Autodesk Inventor part; units mm, degrees
ref_plane "YZ Plane" through (0, 0, 0) normal (1, 0, 0) x (0, 1, 0)
ref_plane "XZ Plane" through (0, 0, 0) normal (0, 1, 0) x (-1, 0, 0)
ref_plane "XY Plane" through (0, 0, 0) normal (0, 0, 1) x (1, 0, 0)
sketch "Sketch1" plane through (0, 0, 0) normal (0, 0, 1) x (1, 0, 0)
  line L0 (-6, 110.6647) -> (-6, 110.2647)
  arc A0 (-6, 110.2647) -> (-5.6, 109.8647) centre (-5.6, 110.2647) ccw
  line L1 (-5.6, 109.8647) -> (-4.9, 109.8647)
  arc A1 (-4.9, 109.8647) -> (-4.7, 110.0647) centre (-4.9, 110.0647) ccw
  line L2 (-4.7, 110.0647) -> (-4.7, 110.3147)
  arc A2 (-4.5, 110.5147) -> (-4.7, 110.3147) centre (-4.5, 110.3147) ccw
  line L3 (-4.5, 110.5147) -> (-1.8, 110.5147)
  arc A3 (-1.4, 110.1147) -> (-1.8, 110.5147) centre (-1.8, 110.1147) ccw
  line L4 (-1.4, 110.1147) -> (-1.4, 104.4147)
  line L5 (-1.8, 104.0147) -> (-4.5, 104.0147)
  arc A4 (-1.8, 104.0147) -> (-1.4, 104.4147) centre (-1.8, 104.4147) ccw
  arc A5 (-4.7, 104.2147) -> (-4.5, 104.0147) centre (-4.5, 104.2147) ccw
  line L6 (-4.7, 104.2147) -> (-4.7, 104.4647)
  arc A6 (-4.7, 104.4647) -> (-4.9, 104.6647) centre (-4.9, 104.4647) ccw
  line L7 (-4.9, 104.6647) -> (-5.6, 104.6647)
  arc A7 (-5.6, 104.6647) -> (-6, 104.2647) centre (-5.6, 104.2647) ccw
  line L8 (-6, 104.2647) -> (-6, 103.6647)
  line L9 (-6.5, 116.6647) -> (-6.5, 110.6647)
  line L10 (-6.5, 110.6647) -> (-2.5, 110.6647)
  line L11 (-1.05, 103.6647) -> (-6.5, 103.6647)
  line L12 (-6.5, 103.6647) -> (-6.5, 97.1647)
  line L13 (-6.5, 97.1647) -> (-1.05, 97.1647)
  line L14 (-6, 97.1647) -> (-6, 96.5647)
  arc A8 (-6, 96.5647) -> (-5.6, 96.1647) centre (-5.6, 96.5647) ccw
  line L15 (-5.6, 96.1647) -> (-4.9, 96.1647)
  arc A9 (-4.9, 96.1647) -> (-4.7, 96.3647) centre (-4.9, 96.3647) ccw
  arc A10 (-4.5, 96.8147) -> (-4.7, 96.6147) centre (-4.5, 96.6147) ccw
  line L16 (-4.7, 96.3647) -> (-4.7, 96.6147)
  line L17 (-4.5, 96.8147) -> (-1.8, 96.8147)
  arc A11 (-1.4, 96.4147) -> (-1.8, 96.8147) centre (-1.8, 96.4147) ccw
  line L18 (-1.4, 96.4147) -> (-1.4, 90.7147)
  arc A12 (-1.8, 90.3147) -> (-1.4, 90.7147) centre (-1.8, 90.7147) ccw
  line L19 (-1.8, 90.3147) -> (-4.5, 90.3147)
  arc A13 (-4.7, 90.5147) -> (-4.5, 90.3147) centre (-4.5, 90.5147) ccw
  line L20 (-4.7, 90.5147) -> (-4.7, 90.7647)
  arc A14 (-4.7, 90.7647) -> (-4.9, 90.9647) centre (-4.9, 90.7647) ccw
  line L21 (-4.9, 90.9647) -> (-5.6, 90.9647)
  arc A15 (-5.6, 90.9647) -> (-6, 90.5647) centre (-5.6, 90.5647) ccw
  line L22 (-6, 90.5647) -> (-6, 90.1647)
  line L23 (-2.5, 90.1647) -> (-6.5, 90.1647)
  line L24 (-6.5, 90.1647) -> (-6.5, 84.1647)
  line L25 (32.5, 123.1647) -> (0, 123.1647)
  circle A16 centre (0, 116.6647) radius 4.75
  circle A17 centre (32.5, 116.6647) radius 4.75
  circle A18 centre (0, 84.1647) radius 4.75
  circle A19 centre (32.5, 84.1647) radius 4.75
  line L26 (39, 97.1647) -> (39, 103.6647)
  line L27 (39, 110.6647) -> (39, 116.6647)
  line L28 (39, 84.1647) -> (39, 90.1647)
  line L29 (26.5, 77.6647) -> (32.5, 77.6647)
  line L30 (0, 77.6647) -> (6, 77.6647)
  line L31 (13, 77.6647) -> (19.5, 77.6647)
  circle A20 centre (16.25, 100.4147) radius 15
  circle A21 centre (16.2588, 5.0016) radius 2.5
  circle A22 centre (16.25, -50.5) radius 2.5
  circle A23 centre (16.25, 100.4147) radius 5
  circle A24 centre (16.25, 100.4147) radius 8.45
  line L32 (24.75, 95.5072) -> (24.75, 105.3221)
  line L33 (44, 10) -> (-11.5, 10)
  line L34 (-11.5, 10) -> (-11.5, -55.5)
  line L35 (-11.5, -55.5) -> (44, -55.5)
  line L36 (44, -55.5) -> (44, 10)
  line L37 (-11.5, 30) -> (44, 30)
  line L38 (-11.5, -75.5) -> (-11.5, 30)
  line L39 (44, 30) -> (44, -75.5)
  line L40 (44, -75.5) -> (-11.5, -75.5)
  circle A25 centre (16.25, -65.5) radius 5
  circle A26 centre (16.25, 20) radius 5
  line L41 (-11.5, 37.6647) -> (44, 37.6647)
  line L42 (44, 37.6647) -> (44, 163.1647)
  line L43 (44, 163.1647) -> (-11.5, 163.1647)
  line L44 (-11.5, 163.1647) -> (-11.5, 37.6647)
  line L45 (-11.5, 163.1647) -> (44, 37.6647)
  line L46 (16.25, 100.4147) -> (112.1111, 100.4147)
  dimension "d2" = 125.5
extrude "Extrusion1" add sketch "Sketch1" along normal blind 10 contours L46 A24 L45 A20 | L46 L42 L45 A20 | A20 L45 A24 L46 | A20 L45 L43 L42 L46 | L45 A24 A20 | A20 L45 L41 L44 | L45 A23 A24 | A24 L46 A23 L45 | L45 A23 L46 A24 | L45 A23 | A23 L46 L45 | L45 L46 A23
sketch "Sketch2" plane through (0, 0, 10) normal (0, 0, 1) x (1, 0, 0)
  line L0 (44, 163.1647) -> (-11.5, 163.1647)
  line L1 (44, 37.6647) -> (44, 163.1647)
  line L2 (-11.5, 163.1647) -> (44, 163.1647)
  line L3 (44, 163.1647) -> (44, 153.1647)
  line L4 (44, 153.1647) -> (-11.5, 153.1647)
  line L5 (-11.5, 153.1647) -> (-11.5, 163.1647)
  line L6 (-11.5, 37.6647) -> (44, 37.6647)
  line L7 (44, 37.6647) -> (44, 47.6647)
  line L8 (44, 47.6647) -> (-11.5, 47.6647)
  line L9 (-11.5, 47.6647) -> (-11.5, 37.6647)
  point P0 (0, 0)
  dimension "d5" = 10
  dimension "d6" = 10
extrude "Extrusion2" add sketch "Sketch2" along normal blind 65.5
sketch "Sketch3" plane through (-11.5, 163.1647, 0) normal (0, 1, 0) x (1, 0, 0)
  line L0 (0, -10) -> (55.5, -10)
  line L1 (0, -10) -> (0, -75.5)
  line L2 (55.5, -10) -> (0, -10)
  line L3 (0, -10) -> (0, -75.5)
  line L4 (0, -75.5) -> (55.5, -75.5)
  line L5 (55.5, -75.5) -> (55.5, -10)
  line L6 (55.5, -10) -> (55.5, -75.5)
  line L7 (55.5, -42.75) -> (0, -42.75)
  line L8 (55.5, -10) -> (0, -42.75)
  line L9 (27.75, -26.375) -> (27.75, -42.75)
  line L10 (55.5, -42.75) -> (0, -75.5)
  line L11 (27.75, -59.125) -> (27.75, -42.75)
  circle A0 centre (27.75, -26.375) radius 5
  circle A1 centre (27.75, -59.125) radius 5
  point P0 (11.5, 0)
  dimension "d9" = 10
  dimension "d10" = 10
extrude "Extrusion3" cut sketch "Sketch3" against normal through all contours A0 L9 L8 | L8 A0 | L8 L9 A0 | A1 L10 | L10 L11 A1 | A1 L11 L10
properties part number "AcopleActuadorCarro"
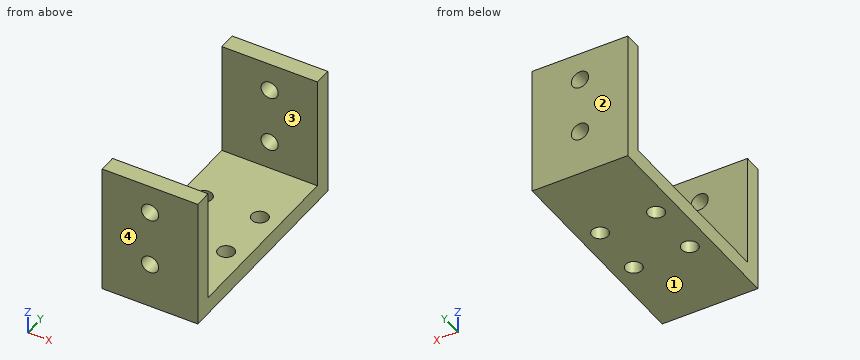
Model file for the job. Use its own axes, mm. Face numbers are marked on the shaded views. Coordinates: 2 decimals unless noted, no trailing zeros. Loops run counter-clockwise (first coordinate to the right, second up) from the corner with the lowest first, then second, coordinate; pieces in that order, holes last. Notation, with made-up numbers: (45.5, 5) -> (56.5, 5) arc R15 ccw to (56.5, 27) -> close; hole circle Ø1 at (61.25, 64.5). An arc over 180 degrees is marked (long way). Use one line per item in the form item = value. Start each with the question number.
(1) Cut at C-C on x = 32.5. Give the cut face in (y, z).
(2) Probe probe 1 along Z at (x, y) = (16.25, 40) (3 decimals); probe 2 along Y at (x, z) = (26, 63); probe 3 along Z at (x, y) = (13.5, 153.5). List the from-to ranges inside material, lowest first. Write a range as from..to.
(3) Cut at A-A on x = 16.25. Give the cut face in (y, z) (3 decimals).
(4) Cut at D-D on z = 57. Give the cut face in (x, y).
(5) Pull direction Y, two halves, no side cores. Call the marked faces 1, 2, 3 and 4: pulls with the +Y half, pulls with the -Y half, needs draft (parallel to the pull), parting line crosses it, or undercut.
(6) Flat gauge pins, fed straight in: pin 1 (1 mm diameter, centred on x = 38.5, y = 98.5, fed in from +Z); pin 2 (7.5 mm diameter, centred on x = 32.5, y = 116.66, fed in from +Z). Where does each tip first touch, or does it go through?
(7) Cut at B-B on z = 67.5. Give the cut face in (x, y), and give its area (3 significant figures).
Values:
q1.outline = (37.66, 0) -> (79.41, 0) -> (79.41, 10) -> (47.66, 10) -> (47.66, 75.5) -> (37.66, 75.5) -> close; (88.91, 0) -> (111.91, 0) -> (111.91, 10) -> (88.91, 10) -> close; (121.41, 0) -> (163.16, 0) -> (163.16, 75.5) -> (153.16, 75.5) -> (153.16, 10) -> (121.41, 10) -> close
q2.probe_1 = 0..21.375, 31.375..54.125, 64.125..75.5
q2.probe_2 = 37.66..47.66, 153.16..163.16
q2.probe_3 = 0..22.2, 30.55..54.95, 63.3..75.5
q3.outline = (37.665, 0) -> (163.165, 0) -> (163.165, 21.375) -> (153.165, 21.375) -> (153.165, 10) -> (47.665, 10) -> (47.665, 21.375) -> (37.665, 21.375) -> close; (37.665, 31.375) -> (47.665, 31.375) -> (47.665, 54.125) -> (37.665, 54.125) -> close; (37.665, 64.125) -> (47.665, 64.125) -> (47.665, 75.5) -> (37.665, 75.5) -> close; (153.165, 31.375) -> (163.165, 31.375) -> (163.165, 54.125) -> (153.165, 54.125) -> close; (153.165, 64.125) -> (163.165, 64.125) -> (163.165, 75.5) -> (153.165, 75.5) -> close
q4.outline = (-11.5, 37.66) -> (11.72, 37.66) -> (11.72, 47.66) -> (-11.5, 47.66) -> close; (-11.5, 153.16) -> (11.72, 153.16) -> (11.72, 163.16) -> (-11.5, 163.16) -> close; (20.78, 37.66) -> (44, 37.66) -> (44, 47.66) -> (20.78, 47.66) -> close; (20.78, 153.16) -> (44, 153.16) -> (44, 163.16) -> (20.78, 163.16) -> close
q5.face_1 = needs draft
q5.face_2 = pulls with the +Y half
q5.face_3 = undercut
q5.face_4 = pulls with the -Y half
q6.pin_1 = 10
q6.pin_2 = through
q7.outline = (-11.5, 37.66) -> (44, 37.66) -> (44, 47.66) -> (-11.5, 47.66) -> close; (-11.5, 153.16) -> (44, 153.16) -> (44, 163.16) -> (-11.5, 163.16) -> close
q7.area = 1,110 mm2
